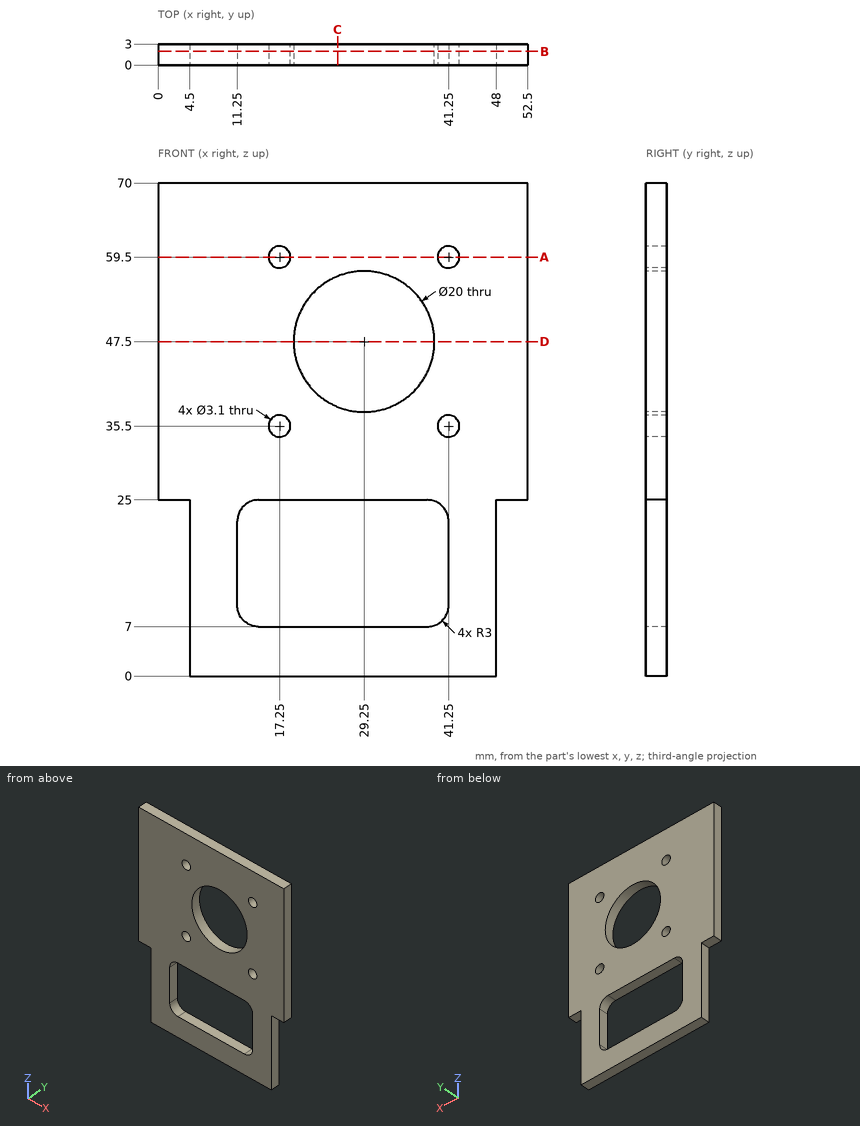
Design review of the part shown in the three views and the two pictorial views. Dimensions are in mm from the part's minimum x, y and z. Coordinates: 2 decimals unless noted, no trailing zeros. Order: outer loops, then holes, each group sorted by start corner. A loop starts at its lowest first (then second) coordinate and runs counter-clockwise, first axis right, second up.
Item 1: For pin 1 Ø0.9 at (y, z) = (1.5, 18) entering from +X; pin 2 Ø0.9 at (y, z) = (2, 13.5) entering from -X, all flat-tipped, find the tip position at first contact; note any pin that passes through.
Item 2: Take a section at C-C, the plane x = 25.5. Write out the cut boundary in (y, z).
Item 3: Take a section at D-D, the plane z = 47.5. Write out the cut boundary in (x, y), then the cut area to 3 significant figures.
Item 4: For line 1 (Z direction, x = 17.25, y = 1.5); line 2 (Z direction, x = 29.25, y = 1.85); line 3 (X direction, y = 0.4, z = 48), list the stretches that pass through material, from the lowest coordinate up.
Item 5: Take a section at B-B, the plane y = 1.95. Write out the cut boundary in (x, z).
Item 6: Take a section at A-A, the plane z = 59.5. Write out the cut boundary in (x, y).
The answers:
1. pin 1: stops at x = 48
1. pin 2: stops at x = 4.5
2. outline: (0, 0) - (3, 0) - (3, 7) - (0, 7) - close; (0, 25) - (3, 25) - (3, 38.23) - (0, 38.23) - close; (0, 56.77) - (3, 56.77) - (3, 70) - (0, 70) - close
3. outline: (0, 0) - (19.25, 0) - (19.25, 3) - (0, 3) - close; (39.25, 0) - (52.5, 0) - (52.5, 3) - (39.25, 3) - close
3. area: 97.5 mm2
4. line 1: z = 0 to 7, 25 to 33.95, 37.05 to 57.95, 61.05 to 70
4. line 2: z = 0 to 7, 25 to 37.5, 57.5 to 70
4. line 3: x = 0 to 19.26, 39.24 to 52.5
5. outline: (0, 25) - (4.5, 25) - (4.5, 0) - (48, 0) - (48, 25) - (52.5, 25) - (52.5, 70) - (0, 70) - close; hole (11.25, 10) arc R3 ccw to (14.25, 7) - (38.25, 7) arc R3 ccw to (41.25, 10) - (41.25, 22) arc R3 ccw to (38.25, 25) - (14.25, 25) arc R3 ccw to (11.25, 22) - close; hole circle Ø3.1 at (17.25, 35.5); hole circle Ø3.1 at (17.25, 59.5); hole circle Ø20 at (29.25, 47.5); hole circle Ø3.1 at (41.25, 35.5); hole circle Ø3.1 at (41.25, 59.5)
6. outline: (0, 0) - (15.7, 0) - (15.7, 3) - (0, 3) - close; (18.8, 0) - (39.7, 0) - (39.7, 3) - (18.8, 3) - close; (42.8, 0) - (52.5, 0) - (52.5, 3) - (42.8, 3) - close
